Read the model definition and answer for the solid it produces. Units are mm, in the model's axes. A direction names the side the tool comes from. Coordinates: 2 decimals unless noted, no trailing zeros. Loops run counter-clockwise (first coordinate to the right, second up) from the corner with the lowest first, then second, coordinate; pieces in that order, holes last. Notation, with made-up numbers: (51, -2) -> (57, -2) arc R24 ccw to (57, 21) -> close; hole circle Ø6 at (-18.5, 39). An arc over 180 degrees is marked (long way). Answer as a JSON object with one key per item and string values. Group by question number.
Q1. Straight lines are drawn through the part: line 1 along X through (y, z) = (-11, 5) (3 decimals); line 2 along Z through (x, y) = (0, -2.5); line 3 along Z through (x, y) = (19, 1) (3 decimals). For each, find the intervals that lie inside material, in ascending order. Write a range as [from, to].
Q2. The part is cut by section B-B on z = -12.7. State how many separate pieces and enclosed holes the cut face has, and give its area (3 significant figures).
Q3. Each of these flat-tipped pins is pushed along its axis until it touches: P1, Ø1.2, axis at x = 11.5, y = -11.5, coming from the +Z side; P2, Ø6.5, axis at x = 12.7, z = 29.21, coming from the -Y side; P3, Ø4, axis at x = -2, y = 3, coming from the -Z side. Where does it stop, or does it pass through?
Q4. Determine the mould class of faces 1 (the flat face through (19.685, 10, -2)), 2 (the cylindrical face through (-0.1, -7.94, -28.71)), 3 (the flat face through (19.094, 2.881, 34.881)) for opening direction Z: released by +Z, released by -Z, zero draft, split by the parting line, or undercut.
Q5. The part is cut by section D-D on z = 29.21. Write down the section's boundary in (x, y) (1 decimal), and give its area (3 significant figures).
Q6. For faces 4 (the flat face through (17, -10, 12.192)), 5 (the flat face through (19.685, 10, 26)), 6 (the cylindrical face through (-11.922, 0.178, -7.305)), 7 (the flat face through (-12.827, 6, -24)), 8 (the cylindrical face through (-16.083, -7.935, 2.735)), determine the directions among +Z, -Z, +X, -X, +Y, -Y from which every point of the face is accessible in a straight line to the end or side of a thin tool.
from build123d import *

# Parameters (mm, degrees)
BASE_DEPTH                    = 12.7
BASE_DEPTH_BACK               = 12.7
SKETCH1_W                     = 44.45
SKETCH1_H                     = 76.2
SKETCH2_R                     = 4.7625
SHAFTGUIDE_DEPTH              = 25.4
ACTUATORPLANECUT_DEPTH        = 6.0325
CENTERSLOT_DEPTH              = 46.900442536
CENTERSLOT_DEPTH_BACK         = 46.900442536
SKETCH5_W                     = 25.654
SKETCH5_H                     = 12.7
CENTERSLOTFILLET_R            = 3.175
GEARBOXPIT_DEPTH              = 11.176
SKETCH60_W                    = 25.654
SKETCH60_H                    = 22.225
FRONTCUTAWAY_DEPTH            = 12.7
CHAMFERFRONT_SIZE             = 9.525
GEARBOXSLOTSH_DEPTH           = 2.286
SKETCH55_R                    = 1.5875
GUIDEBARHOLE_DEPTH            = 60.905780189
PITCHSHAFTHOLE_DEPTH          = 46.900442612
PITCHSHAFTHOLE_DEPTH_BACK     = 46.900442612
SKETCH56_R                    = 3.175
SKETCH57_R                    = 6.35
BEARINGBORER_DEPTH            = 4.064
BEARINGBORESETSCREWS_REACH    = 62.778
BEARINGBORESETSCREWS_BORE_R   = 1.1303
TOGGLEASSEMHOLES_D            = 2.7051
TOGGLEASSEMHOLES_DEPTH        = 9.398
TOGGLEASSEMHOLES_TIP          = 0.81269403
BACKCHAMFERS_SIZE             = 6.35
PITCHMOTORSLOT_DEPTH          = 60.905780284
PITCHMOTORMOUNTINGSLOTS_DEPTH = 2.54
PITCHMOTORMOUNTINGHOLES_D     = 2.2606
PITCHMOTORMOUNTINGHOLES_DEPTH = 7.5946
PITCHMOTORMOUNTINGHOLES_TIP   = 0.679152758
GEARBOXMOUNTINGHOLES_D        = 2.7051
GEARBOXMOUNTINGHOLES_DEPTH    = 9.398
GEARBOXMOUNTINGHOLES_TIP      = 0.81269403
CAPMOUNTINGHOLES_D            = 3.6576
CAPMOUNTINGHOLES_CBORE_D      = 7.14502
CAPMOUNTINGHOLES_CBORE_DEPTH  = 3.5052


with BuildPart() as part:
    # Sketch1 → Base (new, two sides: drawn at the far end of the back side and taken through both)
    with BuildSketch(Plane(origin=(0, 0, 0), x_dir=(1, 0, 0), z_dir=(0, 1, 0)).offset(-BASE_DEPTH_BACK)):
        Rectangle(SKETCH1_W, SKETCH1_H)
    extrude(amount=BASE_DEPTH + BASE_DEPTH_BACK)

    # Sketch2 → ShaftGuide (cut)
    with BuildSketch(Plane(origin=(0, 0, -38.1), x_dir=(-1, 0, 0), z_dir=(0, 0, -1))):
        with Locations((0, -12.7)):
            Circle(SKETCH2_R)
    extrude(amount=-SHAFTGUIDE_DEPTH, mode=Mode.SUBTRACT)

    # Sketch3 → ActuatorPlaneCut (cut)
    with BuildSketch(Plane(origin=(0, -12.7, 0), x_dir=(-1, 0, 0), z_dir=(0, -1, 0))):
        Polygon((10.922, -12.192), (16.002, -12.192), (22.225, -12.192), (22.225, -38.1), (-22.225, -38.1), (-22.225, -12.192), (-10.922, -12.192), (-10.922, 4.572), (10.922, 4.572), align=None)
    extrude(amount=-ACTUATORPLANECUT_DEPTH, mode=Mode.SUBTRACT)

    # Sketch5 → CenterSlot (cut, two sides: drawn at the far end of the back side and taken through both)
    with BuildSketch(Plane(origin=(0, 0, 0), x_dir=(1, 0, 0), z_dir=(0, 1, 0)).offset(-CENTERSLOT_DEPTH_BACK)):
        with Locations((0, 12.7)):
            Rectangle(SKETCH5_W, SKETCH5_H)
    extrude(amount=CENTERSLOT_DEPTH + CENTERSLOT_DEPTH_BACK, mode=Mode.SUBTRACT)

    # CenterSlotFillet
    centerslotfillet_edges = [part.edges().sort_by_distance(p)[0] for p in [
        (12.827, 0, -19.05),
        (-12.827, 0, -19.05),
        (-12.827, 0, -6.35),
        (12.827, 0, -6.35),
    ]]
    fillet(centerslotfillet_edges, radius=CENTERSLOTFILLET_R)

    # Sketch40 → GearBoxPit (cut)
    with BuildSketch(Plane.XZ.offset(12.7)):
        with BuildLine():
            Line((10.922, -8.89), (-10.922, -8.89))
            Line((-10.922, -8.89), (-10.922, 9.017))
            ThreePointArc((-10.922, 9.017), (-9.99206403, 11.26206403), (-7.747, 12.192))
            Line((-7.747, 12.192), (7.747, 12.192))
            ThreePointArc((7.747, 12.192), (9.99206403, 11.26206403), (10.922, 9.017))
            Line((10.922, 9.017), (10.922, -8.89))
        make_face()
    extrude(amount=-GEARBOXPIT_DEPTH, mode=Mode.SUBTRACT)

    # Sketch60 → FrontCutaway (cut)
    with BuildSketch(Plane(origin=(0, 12.7, 0), x_dir=(1, 0, 0), z_dir=(0, 1, 0))):
        with Locations((0, 26.9875)):
            Rectangle(SKETCH60_W, SKETCH60_H)
    extrude(amount=-FRONTCUTAWAY_DEPTH, mode=Mode.SUBTRACT)

    # ChamferFront
    chamferfront_edges = [part.edges().sort_by_distance(p)[0] for p in [
        (17.526, 12.7, -38.1),
        (-17.526, 12.7, -38.1),
    ]]
    chamfer(chamferfront_edges, length=CHAMFERFRONT_SIZE)

    # Sketch67 → GearBoxSlotsH (cut)
    with BuildSketch(Plane(origin=(0, -12.7, 0), x_dir=(-1, 0, 0), z_dir=(0, -1, 0))):
        with BuildLine():
            Line((-12.3825, 2.936875), (12.3825, 2.936875))
            ThreePointArc((12.3825, 2.936875), (12.779375, 2.54), (12.3825, 2.143125))
            Line((12.3825, 2.143125), (-12.3825, 2.143125))
            ThreePointArc((-12.3825, 2.143125), (-12.779375, 2.54), (-12.3825, 2.936875))
        make_face()
        with BuildLine():
            Line((-12.3825, -7.731125), (12.3825, -7.731125))
            ThreePointArc((12.3825, -7.731125), (12.779375, -8.128), (12.3825, -8.524875))
            Line((12.3825, -8.524875), (-12.3825, -8.524875))
            ThreePointArc((-12.3825, -8.524875), (-12.779375, -8.128), (-12.3825, -7.731125))
        make_face()
    extrude(amount=-GEARBOXSLOTSH_DEPTH, mode=Mode.SUBTRACT)

    # Sketch55 → GuideBarHole (cut, through all)
    with BuildSketch(Plane.ZY.offset(22.225)):
        with Locations((-17.4625, -9.525)):
            Circle(SKETCH55_R)
    extrude(amount=-GUIDEBARHOLE_DEPTH, mode=Mode.SUBTRACT)

    # Sketch56 → PitchShaftHole (cut, two sides: drawn at the far end of the back side and taken through both)
    with BuildSketch(Plane(origin=(0, 0, 0), x_dir=(0, 0, -1), z_dir=(1, 0, 0)).offset(-PITCHSHAFTHOLE_DEPTH_BACK)):
        with Locations((12.7, 0)):
            Circle(SKETCH56_R)
    extrude(amount=PITCHSHAFTHOLE_DEPTH + PITCHSHAFTHOLE_DEPTH_BACK, mode=Mode.SUBTRACT)

    # Sketch57 → BearingBoreR (cut)
    with BuildSketch(Plane.ZY.offset(22.225)):
        with Locations((-12.7, 0)):
            Circle(SKETCH57_R)
    bearingborer = extrude(amount=-BEARINGBORER_DEPTH, mode=Mode.SUBTRACT)

    # BearingBoreL: BearingBoreR across plane
    add(bearingborer.mirror(Plane(origin=(0, 0, 0), x_dir=(0, 0, 1), z_dir=(1, 0, 0))), mode=Mode.SUBTRACT)

    # BearingBoreSetScrews bore → BearingBoreSetScrews (cut, up to next)
    with BuildSketch(Plane(origin=(4.343261145, 12.7, -10.30436568), x_dir=(1, 0, 0), z_dir=(0, 1, 0)), mode=Mode.PRIVATE) as bearingboresetscrews_sk1:
        with Locations((-24.536261145, 2.39563432)):
            Circle(BEARINGBORESETSCREWS_BORE_R)
    bearingboresetscrews_tool1 = extrude(bearingboresetscrews_sk1.sketch, amount=-BEARINGBORESETSCREWS_REACH, mode=Mode.PRIVATE) & part.part
    # BearingBoreSetScrews bore → BearingBoreSetScrews (cut, up to next)
    with BuildSketch(Plane(origin=(4.343261145, 12.7, -10.30436568), x_dir=(1, 0, 0), z_dir=(0, 1, 0)), mode=Mode.PRIVATE) as bearingboresetscrews_sk2:
        with Locations((15.849738855, 2.39563432)):
            Circle(BEARINGBORESETSCREWS_BORE_R)
    bearingboresetscrews_tool2 = extrude(bearingboresetscrews_sk2.sketch, amount=-BEARINGBORESETSCREWS_REACH, mode=Mode.PRIVATE) & part.part
    add(bearingboresetscrews_tool1.solids().sort_by_distance((-20.193, 12.7, -12.7))[0], mode=Mode.SUBTRACT)
    add(bearingboresetscrews_tool2.solids().sort_by_distance((20.193, 12.7, -12.7))[0], mode=Mode.SUBTRACT)

    # ToggleAssemHoles
    with Locations(Plane(origin=(0, -12.7, 0), x_dir=(-1, 0, 0), z_dir=(0, -1, 0))):
        with Locations((12.7, 31.75), (-12.7, 31.75)):
            Hole(TOGGLEASSEMHOLES_D / 2, depth=TOGGLEASSEMHOLES_DEPTH)
            with Locations((0, 0, -(TOGGLEASSEMHOLES_DEPTH + TOGGLEASSEMHOLES_TIP / 2))):  # 118° drill point
                Cone(0, TOGGLEASSEMHOLES_D / 2, TOGGLEASSEMHOLES_TIP, mode=Mode.SUBTRACT)

    # BackChamfers
    backchamfers_edges = [part.edges().sort_by_distance(p)[0] for p in [
        (-22.225, 3.01625, 38.1),
        (22.225, 3.01625, 38.1),
    ]]
    chamfer(backchamfers_edges, length=BACKCHAMFERS_SIZE)

    # Sketch62 → PitchMotorSlot (cut, through all)
    with BuildSketch(Plane.ZY.offset(22.225)):
        with BuildLine():
            Line((1.905, 9.525), (1.905, 12.7))
            Line((1.905, 12.7), (22.225, 12.7))
            Line((22.225, 12.7), (22.225, 9.525))
            ThreePointArc((22.225, 9.525), (12.065, -0.635), (1.905, 9.525))
        make_face()
    extrude(amount=-PITCHMOTORSLOT_DEPTH, mode=Mode.SUBTRACT)

    # Sketch63 → PitchMotorMountingSlots (cut)
    with BuildSketch(Plane.ZY.offset(-22.225)):
        with BuildLine():
            Line((-3.556, 12.7), (27.686, 12.7))
            Line((27.686, 12.7), (27.686, 9.525))
            ThreePointArc((27.686, 9.525), (26.75606403, 7.27993597), (24.511, 6.35))
            Line((24.511, 6.35), (-0.381, 6.35))
            ThreePointArc((-0.381, 6.35), (-2.62606403, 7.27993597), (-3.556, 9.525))
            Line((-3.556, 9.525), (-3.556, 12.7))
        make_face()
    extrude(amount=PITCHMOTORMOUNTINGSLOTS_DEPTH, mode=Mode.SUBTRACT)

    # PitchMotorMountingHoles
    with Locations(Plane(origin=(19.685, 0, 0), x_dir=(0, 0, -1), z_dir=(1, 0, 0))):
        with Locations((-24.5618, 9.525), (0.4318, 9.525)):
            Hole(PITCHMOTORMOUNTINGHOLES_D / 2, depth=PITCHMOTORMOUNTINGHOLES_DEPTH)
            with Locations((0, 0, -(PITCHMOTORMOUNTINGHOLES_DEPTH + PITCHMOTORMOUNTINGHOLES_TIP / 2))):  # 118° drill point
                Cone(0, PITCHMOTORMOUNTINGHOLES_D / 2, PITCHMOTORMOUNTINGHOLES_TIP, mode=Mode.SUBTRACT)

    # GearBoxMountingHoles
    with Locations(Plane(origin=(0, -12.7, 0), x_dir=(-1, 0, 0), z_dir=(0, -1, 0))):
        with Locations((-14.732, -2.794), (14.732, -2.794)):
            Hole(GEARBOXMOUNTINGHOLES_D / 2, depth=GEARBOXMOUNTINGHOLES_DEPTH)
            with Locations((0, 0, -(GEARBOXMOUNTINGHOLES_DEPTH + GEARBOXMOUNTINGHOLES_TIP / 2))):  # 118° drill point
                Cone(0, GEARBOXMOUNTINGHOLES_D / 2, GEARBOXMOUNTINGHOLES_TIP, mode=Mode.SUBTRACT)

    # CapMountingHoles (through all)
    with Locations(Plane(origin=(-0.837932951, 12.7, 8.633720573), x_dir=(-1, 0, 0), z_dir=(0, 1, 0))):
        with Locations((-13.537932951, 20.576279427), (11.862067049, 20.576279427)):
            CounterBoreHole(CAPMOUNTINGHOLES_D / 2, CAPMOUNTINGHOLES_CBORE_D / 2, CAPMOUNTINGHOLES_CBORE_DEPTH)


solid = part.part
Final values:
{
 "1": {"line 1": "x = [-22.225, -10.922], [10.922, 22.225]", "line 2": "z = [-38.1, -19.05], [12.19, 38.1]", "line 3": "z = [-38.1, -18.971], [-6.429, 6.538], [17.592, 34.975]"},
 "2": {"separate pieces": "6", "enclosed holes": "0", "area": "278 mm2"},
 "3": {"P1": "stops at z = 12.19", "P2": "stops at y = -6.67", "P3": "stops at z = -6.35"},
 "4": {"face 1": "undercut", "face 2": "zero draft", "face 3": "released by +Z"},
 "5": {"outline": "(-22.2, -6.7) -> (-14.5, -6.7) -> (-14.5, 9.2) -> (-16.3, 9.2) -> (-16.3, 12.7) -> (-22.2, 12.7) -> close; (-10.9, -6.7) -> (10.9, -6.7) -> (10.9, 9.2) -> (9.1, 9.2) -> (9.1, 12.7) -> (-9.1, 12.7) -> (-9.1, 9.2) -> (-10.9, 9.2) -> close; (14.5, -6.7) -> (22.2, -6.7) -> (22.2, 12.7) -> (16.3, 12.7) -> (16.3, 9.2) -> (14.5, 9.2) -> close", "area": "695 mm2"},
 "6": {"face 4": "+Z, +X, -X, -Y", "face 5": "+X, +Y", "face 6": "+Y, -Y", "face 7": "-Z, +Y", "face 8": "-Y"}
}
